from build123d import *

# Parameters (mm, degrees)
F0_W     = 25.4
F0_H     = 431.8
F1_DEPTH = 25.4
F2_T     = -2.54
F4_DEPTH = 6.35
F5_R     = 3.2639
F6_DEPTH = 2.54


with BuildPart() as f1:
    # F0 (on Front) → F1 (new body)
    with BuildSketch(Plane.XZ):
        with Locations((12.7, -215.9)):
            Rectangle(F0_W, F0_H)
    extrude(amount=F1_DEPTH)

    # F2
    f2_openings = [f1.faces().sort_by_distance(p)[0] for p in [
        (12.7, -12.7, 0),
        (12.7, -12.7, -431.8),
    ]]
    offset(amount=F2_T, openings=f2_openings)

    # F3 (on face) → F4 (cut)
    with BuildSketch(Plane.XZ.offset(25.4)):
        with BuildLine():
            Line((19.05, -279.4), (19.05, -25.4))
            ThreePointArc((19.05, -25.4), (12.7, -19.05), (6.35, -25.4))
            Line((6.35, -25.4), (6.35, -279.4))
            ThreePointArc((6.35, -279.4), (12.7, -285.75), (19.05, -279.4))
        make_face()
    extrude(amount=-F4_DEPTH, mode=Mode.SUBTRACT)

    # F5 (on face) → F6 (cut)
    with BuildSketch(Plane(origin=(0, 0, 0), x_dir=(-1, 0, 0), z_dir=(0, 1, 0))):
        with Locations((-12.7, -25.4)):
            Circle(F5_R)
    extrude(amount=-F6_DEPTH, mode=Mode.SUBTRACT)


solid = f1.part
Read the model definition and answer for the solid it produces. Units are mm, in the model's axes. A direction names the side the tool comes from. Round coordinates to 2 decimals unless told otherwise and drop trailing zeros. Write each loop counter-clockwise with the first axis right and the second up, starting at its lowest first coordinate (ties: lowest second). Pieces come first, ordered by that corner, then holes. Notation, with made-up numbers: (7.25, 81.5) - (35.25, 81.5) arc R13 cw to (35.25, 90.5) - close; hole circle Ø2 at (-5.75, 33). An arc over 180 degrees is marked (long way). One line per question, with ' | ' between items. Start each with the question number.
1. Section C-C (z = -32.5) is taken. Determine the outline of the cut face in (x, y).
2. For a pull along Y with two mould halves and no side action, classify faces 3 (the face through (13, 0, -213)), 4 (the face through (22.86, -13, -219)), 5 (the face through (24, -13, 0)) as +Y half, -Y half, draft (parallel to the pull), parting line (faces both ways), or undercut.
3. Each of these flat-tipped pins is pushed along its axis until it touches: pin 1 (2 mm diameter, centred on x = 20, y = -3.5, fed in from +Z); pin 2 (4 mm diameter, centred on x = 9, z = -216, fed in from -Y). Where does it stop, or does it pass through?
4. For faces 1 (the face through (24, -13, -431.8)), 2 (the face through (13, -2.54, -213)), determine the directions among +Z, -Z, +X, -X, +Y, -Y from which every point of the face is accessible in a straight line to the end or side of a thin tool.
5. Section A-A (y = -9) is taken. Determine the outline of the cut face in (x, z), and give its area (3 significant figures).
6. Find the intervals of material crossed by probe 1 along Z at (x, y) = (12, -23.25); probe 2 along X at (y, z) = (-4.75, -43); probe 3 along Z at (x, y) = (12.7, -1), in increasing order. Write a range as [from, to].
7. Section B-B (z = -332) is taken. Determine the outline of the cut face in (x, y), and give its area (3 significant figures).
Filled in:
1) outline: (0, -25.4) - (6.35, -25.4) - (6.35, -22.86) - (2.54, -22.86) - (2.54, -2.54) - (22.86, -2.54) - (22.86, -22.86) - (19.05, -22.86) - (19.05, -25.4) - (25.4, -25.4) - (25.4, 0) - (0, 0) - close
2) face 3: +Y half | face 4: undercut | face 5: draft
3) pin 1: z = 0 | pin 2: y = -2.54
4) face 1: -Z, +X, -X, +Y, -Y | face 2: +Z, -Z
5) outline: (0, -431.8) - (2.54, -431.8) - (2.54, 0) - (0, 0) - close; (22.86, -431.8) - (25.4, -431.8) - (25.4, 0) - (22.86, 0) - close | area: 2,190 mm²
6) probe 1: [-431.8, -285.71], [-19.09, 0] | probe 2: [0, 2.54], [22.86, 25.4] | probe 3: [-431.8, -28.66], [-22.14, 0]
7) outline: (0, -25.4) - (25.4, -25.4) - (25.4, 0) - (0, 0) - close; hole (2.54, -22.86) - (22.86, -22.86) - (22.86, -2.54) - (2.54, -2.54) - close | area: 232 mm²
